```python
from build123d import *

# Parameters (mm, degrees)
SKETCH7_R          = 2.75
CUT_EXTRUDE3_DEPTH = 11.926156548


with BuildPart() as part:
    # Sketch2 → Revolve2 (revolve)
    with BuildSketch(Plane(origin=(0, 0, 0), x_dir=(0, 0, -1), z_dir=(1, 0, 0))):
        Polygon((-0.541748287, -1.269840707), (6.851295576, -1.269840707), (6.851295576, 1.28177138), (6.851295576, 2.78177138), (3.137110203, 2.486943896), (3.137110203, 1.279043896), (3.137110203, 2.779043896), (-0.541748287, 2.475013223), (-0.541748287, 1.267113223), (-0.541748287, 2.767113223), (-4.074860971, 2.475127372), (-4.074860971, 0.975127372), (-4.074860971, -1.269840707), align=None)
    revolve(axis=Axis((0, -1.269840707, 0.541748287), (0, 0, -1)))

    # Sketch7 → Cut-Extrude3 (cut, through all)
    with BuildSketch(Plane(origin=(0, 0, -6.851295576), x_dir=(-1, 0, 0), z_dir=(0, 0, -1))):
        with Locations((0, -1.269840707)):
            Circle(SKETCH7_R)
    extrude(amount=-CUT_EXTRUDE3_DEPTH, mode=Mode.SUBTRACT)


solid = part.part
```
Input: part model. Units: mm. Frame: model coordinates. A direction names the side the tool comes from. Give positions to 0.01 mm unless a question says otherwise; leave off trailing zeros. Loops run counter-clockwise (first coordinate to the right, second up) from the corner with the lowest first, then second, coordinate; pieces in that order, holes last.
1) Section query C-C on z = 2.5. Return the cut outline in (x, y).
A:
outline: circle Ø7.75 at (0, -1.27); hole circle Ø5.5 at (0, -1.27)
2) Line query: L1, parallel to Y at x = 0, z = -0.5; L2, parallel to X at y = -2, z = -3.25; L3, parallel to X at y = -3, z = -4.5. Output: solid intervals per line, ascending.
A:
L1: y = -5.1 to -4.02, 1.48 to 2.56
L2: x = -3.69 to -2.65, 2.65 to 3.69
L3: x = -3.46 to -2.14, 2.14 to 3.46
3) Mould query, pull axis Z, two halves, no side actions, for faces 3 (the flat face through (3, -1, 4.075)), 4 (the conical face through (-2.349, -4.334, -0.863)), 5 (the flat face through (-3, -2, -6.851)). Classes: released by +Z, released by -Z, zero draft, split by the parting line, or undercut.
A:
face 3: released by +Z
face 4: undercut
face 5: released by -Z
4) Section query A-A on x = 0. Return the cut outline in (y, z).
A:
outline: (-5.32, -6.85) - (-4.02, -6.85) - (-4.02, 4.07) - (-5.01, 4.07) - (-5.31, 0.54) - (-5.01, 0.54) - (-5.32, -3.14) - (-5.03, -3.14) - close; (1.48, -6.85) - (2.78, -6.85) - (2.49, -3.14) - (2.78, -3.14) - (2.48, 0.54) - (2.77, 0.54) - (2.48, 4.07) - (1.48, 4.07) - close
5) Reachability of faces 1 (the conical face through (0.17, -5.135, -4.556)), 2 (the cylindrical face through (2.182, -2.943, -1.465)) from +Z, -Z, +X, -X, +Y, -Y: full face, straight path, thin tool, end or side. Return the list, or none.
A:
face 1: none
face 2: +Z, -Z
6) Contact query for flat-ended pins moving along their axis: pin 1 (3 mm diameter, centred on x = -2, z = -2.5, fed in from -Y); pin 2 (1.5 mm diameter, centred on y = -2.5, z = -2.5, fed in from +X); pin 3 (3 mm diameter, centred on x = -3, z = -0.5, fed in from +Y). Output: stop coordinate, or through.
A:
pin 1: stops at y = -5.27
pin 2: stops at x = 3.99
pin 3: stops at y = 2.28
7) Section query B-B on z = 0.75. Return the cut outline in (x, y).
A:
outline: circle Ø8.04 at (0, -1.27); hole circle Ø5.5 at (0, -1.27)
